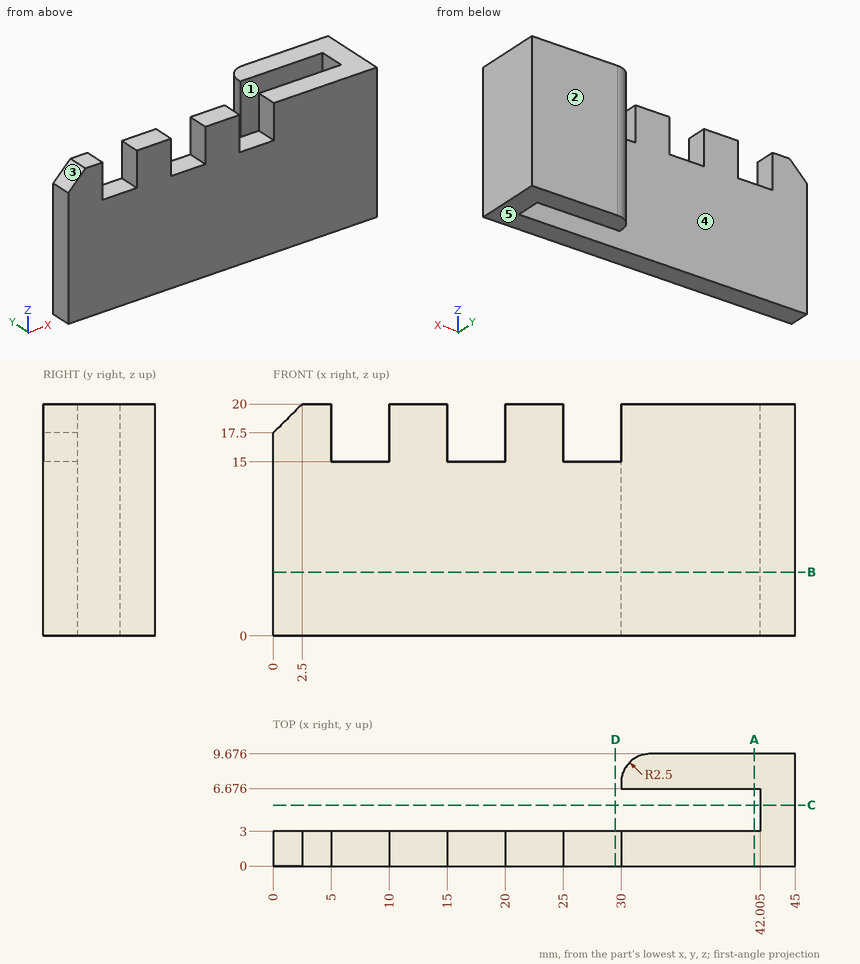
Study the drawing (mm; zero at the part's minimum x, y, z) and answer. A direction names the side the tool comes from. Give positions to 0.01 mm unless a question says otherwise; leave off trailing zeros. Loops run counter-clockwise (first coordinate to the right, second up) from the corner with the lowest first, then second, coordinate; pieces in that order, holes last. Notation, with made-up numbers: M 61.25,62 L 104.25,62 A36 cw 104.25,101 Z; hole C 83,68.5 d9. An arc over 180 degrees is marked long. Answer as CSV lines item,"result".
Item 1: Which of the six approach directions +Z, -Z, +X, -X, +Y, -Y give full straight-line access (tool end or side, diameter ignored) to the marked faces 4 and 5?
Values follow:
face 4,"+Z, -Z, -X"
face 5,"-Z, +X, -X, +Y, -Y"
Item 2: The part is cut by section A-A (x = 41.5). Give the vertices of the cut face in (y, z).
Values follow:
outline,"M 0,0 L 3,0 L 3,20 L 0,20 Z; M 6.68,0 L 9.68,0 L 9.68,20 L 6.68,20 Z"
Item 3: The mould has two halves that part along Y. Classify the marked faces 1, 2 and 3: released by +Y, released by -Y, zero draft, split by the parting line, or undercut.
Values follow:
face 1,"undercut"
face 2,"released by +Y"
face 3,"zero draft"
Item 4: Given pin 1 Ø3.5 at (x, y) = (7, 1) entering from +Z; pin 2 Ø4 at (y, z) = (5.5, 11) entering from -X; pin 3 Ø10 at (x, z) = (17.5, 12) entering from +Y, each flat-ended and moving along its own axis, determine where each tip first touches the part or whether it passes through.
Values follow:
pin 1,"stops at z = 15"
pin 2,"stops at x = 30"
pin 3,"stops at y = 3"
Item 5: The part is cut by section B-B (z = 5.5). Give the vertices of the cut face in (x, y) (1 decimal).
Values follow:
outline,"M 0,0 L 45,0 L 45,9.7 L 32.5,9.7 A2.5 ccw 30,7.2 L 30,6.7 L 42,6.7 L 42,3 L 0,3 Z"
Item 6: The part is cut by section C-C (y = 5.25). Give the vertices of the cut face in (x, z) (1 decimal).
Values follow:
outline,"M 42,0 L 45,0 L 45,20 L 42,20 Z"
Item 7: The part is cut by section D-D (x = 29.5). Give the vertices of the cut face in (y, z).
Values follow:
outline,"M 0,0 L 3,0 L 3,15 L 0,15 Z"
Item 8: Straight lines are drawn through the part: line 1 along Y through (x, z) = (35.5, 3); line 2 along X through (y, z) = (2.75, 18.25); line 3 along Y through (x, z) = (24.5, 5). For each, find the intervals that lie inside material, in ascending order. Write a range as [from, to].
Values follow:
line 1,"y = [0, 3], [6.68, 9.68]"
line 2,"x = [0.75, 5], [10, 15], [20, 25], [30, 45]"
line 3,"y = [0, 3]"
